Can you work these out from the model? Positions are in its coordinate system, mm. A direction names the side the tool comes from. Give positions to 0.01 mm unless a question says otherwise; leave off trailing zeros. Loops run counter-clockwise (first coordinate to the right, second up) from the corner with the lowest first, then second, coordinate; pieces in that order, holes last.
from build123d import *

# Parameters (mm, degrees)
CYLINDER870_R               = 1.5
CYLINDER870_DEPTH           = 20
CYLINDER865_R               = 1.5
CYLINDER865_DEPTH           = 20
CYLINDER862_R               = 1.5
CYLINDER862_DEPTH           = 20
CYLINDER868_R               = 1.5
CYLINDER868_DEPTH           = 20
BOX131_W                    = 6
BOX131_H                    = 2
BOX131_DEPTH                = 6
BOX130_W                    = 6
BOX130_H                    = 2
BOX130_DEPTH                = 6
BOX133_W                    = 6
BOX133_H                    = 2
BOX133_DEPTH                = 6
BOX132_W                    = 6
BOX132_H                    = 2
BOX132_DEPTH                = 6
CYLINDER872_R               = 4
CYLINDER872_DEPTH           = 20
CYLINDER872_PLACEMENT_ANGLE = 45
CYLINDER871_R               = 4
CYLINDER871_DEPTH           = 20
CYLINDER871_PLACEMENT_ANGLE = 45
CYLINDER863_R               = 10
CYLINDER863_DEPTH           = 40
CYLINDER908_R               = 10
CYLINDER908_DEPTH           = 40
CYLINDER864_R               = 52
CYLINDER864_DEPTH           = 10
BOX129_W                    = 108
BOX129_H                    = 36
BOX129_DEPTH                = 10
FILLET013_R                 = 12


with BuildPart() as obj1:
    # Cylinder870 → Cylinder870 (new body)
    with BuildSketch(Plane(origin=(20, -40, -5), x_dir=(1, 0, 0), z_dir=(0, -1, 0))):
        Circle(CYLINDER870_R)
    extrude(amount=CYLINDER870_DEPTH)


with BuildPart() as obj2:
    # Cylinder865 → Cylinder865 (new body)
    with BuildSketch(Plane(origin=(51, -40, 7), x_dir=(1, 0, 0), z_dir=(0, -1, 0))):
        Circle(CYLINDER865_R)
    extrude(amount=CYLINDER865_DEPTH)


with BuildPart() as obj3:
    # Cylinder862 → Cylinder862 (new body)
    with BuildSketch(Plane(origin=(-51, -40, 7), x_dir=(1, 0, 0), z_dir=(0, -1, 0))):
        Circle(CYLINDER862_R)
    extrude(amount=CYLINDER862_DEPTH)


with BuildPart() as compound261:
    # Cylinder868 → Cylinder868 (new body)
    with BuildSketch(Plane(origin=(-20, -40, -5), x_dir=(1, 0, 0), z_dir=(0, -1, 0))):
        Circle(CYLINDER868_R)
    extrude(amount=CYLINDER868_DEPTH)

    # Compound261: union obj1, obj2, obj3
    add(obj1.part)
    add(obj2.part)
    add(obj3.part)


with BuildPart() as krychle131:
    # Box131 → Box131 (new body)
    with BuildSketch(Plane(origin=(17, -47, -8), x_dir=(1, 0, 0), z_dir=(0, 0, 1))):
        with Locations((3, 1)):
            Rectangle(BOX131_W, BOX131_H)
    extrude(amount=BOX131_DEPTH)


with BuildPart() as krychle130:
    # Box130 → Box130 (new body)
    with BuildSketch(Plane(origin=(48, -45, 4), x_dir=(1, 0, 0), z_dir=(0, 0, 1))):
        with Locations((3, 1)):
            Rectangle(BOX130_W, BOX130_H)
    extrude(amount=BOX130_DEPTH)


with BuildPart() as krychle133:
    # Box133 → Box133 (new body)
    with BuildSketch(Plane(origin=(-54, -45, 4), x_dir=(1, 0, 0), z_dir=(0, 0, 1))):
        with Locations((3, 1)):
            Rectangle(BOX133_W, BOX133_H)
    extrude(amount=BOX133_DEPTH)


with BuildPart() as compound258:
    # Box132 → Box132 (new body)
    with BuildSketch(Plane(origin=(-23, -47, -8), x_dir=(1, 0, 0), z_dir=(0, 0, 1))):
        with Locations((3, 1)):
            Rectangle(BOX132_W, BOX132_H)
    extrude(amount=BOX132_DEPTH)

    # Compound258: union Krychle131, Krychle130, Krychle133
    add(krychle131.part)
    add(krychle130.part)
    add(krychle133.part)


with BuildPart() as obj4:
    # Cylinder872 → Cylinder872 (new body)
    with BuildSketch(Plane.XY):
        Circle(CYLINDER872_R)
    extrude(amount=CYLINDER872_DEPTH)


with BuildPart() as obj4_1:
    # Cylinder872 placement: moved
    add(obj4.part.moved(Location((39.6, -39.6, -10))).rotate(Axis((39.6, -39.6, -10), (0, 0, 1)), CYLINDER872_PLACEMENT_ANGLE))


with BuildPart() as compound259:
    # Cylinder871 → Cylinder871 (new body)
    with BuildSketch(Plane.XY):
        Circle(CYLINDER871_R)
    extrude(amount=CYLINDER871_DEPTH)


with BuildPart() as compound259_1:
    # Cylinder871 placement: moved
    add(compound259.part.moved(Location((-39.6, -39.6, -10))).rotate(Axis((-39.6, -39.6, -10), (0, 0, -1)), CYLINDER871_PLACEMENT_ANGLE))

    # Compound259: union obj4
    add(obj4_1.part)


with BuildPart() as obj5:
    # Cylinder863 → Cylinder863 (new body)
    with BuildSketch(Plane(origin=(-59, -17, 0), x_dir=(1, 0, 0), z_dir=(0, 0, 1))):
        Circle(CYLINDER863_R)
    extrude(amount=CYLINDER863_DEPTH)


with BuildPart() as compound260:
    # Cylinder908 → Cylinder908 (new body)
    with BuildSketch(Plane(origin=(59, -17, 0), x_dir=(1, 0, 0), z_dir=(0, 0, 1))):
        Circle(CYLINDER908_R)
    extrude(amount=CYLINDER908_DEPTH)

    # Compound260: union obj5
    add(obj5.part)


with BuildPart() as obj6:
    # Cylinder864 → Cylinder864 (new body)
    with BuildSketch(Plane.XY.offset(20)):
        Circle(CYLINDER864_R)
    extrude(amount=CYLINDER864_DEPTH)


with BuildPart() as fillet013:
    # Box129 → Box129 (new body)
    with BuildSketch(Plane(origin=(-54, -53, 20), x_dir=(1, 0, 0), z_dir=(0, 0, 1))):
        with Locations((54, 18)):
            Rectangle(BOX129_W, BOX129_H)
    extrude(amount=BOX129_DEPTH)

    # Cut147: cut obj6
    add(obj6.part, mode=Mode.SUBTRACT)


with BuildPart() as fillet013_1:
    # Cut147 placement: moved
    add(fillet013.part.moved(Location((0, 0, -20))))

    # Cut146: cut Compound260
    add(compound260.part, mode=Mode.SUBTRACT)

    # Cut149: cut Compound259
    add(compound259_1.part, mode=Mode.SUBTRACT)

    # Cut148: cut Compound258
    add(compound258.part, mode=Mode.SUBTRACT)

    # Cut150: cut Compound261
    add(compound261.part, mode=Mode.SUBTRACT)

    # Fillet013
    fillet013_edges = [fillet013_1.edges().sort_by_distance(p)[0] for p in [
        (-54, -25.660254, 5),
        (54, -25.660254, 5),
    ]]
    fillet(fillet013_edges, radius=FILLET013_R)


solid = fillet013_1.part
(1) Will these pins go through, and if not, where does the flat tip stop? P1, Ø10.5, axis at x = 39.6, y = -39.6, coming from the -Z side; P2, Ø2.5, axis at x = -51, z = 7, coming from the +Y side; P3, Ø1.5, axis at x = -38.5, z = 1.5, coming from the +Y side; P4, Ø1, axis at y = -44, z = 8, coming from the +X side.
Returned:
P1: stops at z = 0
P2: stops at y = -20.8
P3: stops at y = -34.11
P4: stops at x = 48
(2) Suppose I cut it at A-A on y = -48.5. List the corners of the cut face in (x, z) for me (3 decimals).
Returned:
outline: (-54, 0) - (-18.755, 0) - (-18.755, 10) - (-54, 10) - close; (18.755, 0) - (54, 0) - (54, 10) - (18.755, 10) - close; hole circle Ø3 at (-51, 7); hole circle Ø3 at (51, 7)
(3) Please list where these lines run through material, in increasing order: probe 1 along X at (y, z) = (-39.6, 2.75); probe 2 along X at (y, z) = (-47.5, 7); probe 3 along X at (y, z) = (-21.5, 8.5).
Returned:
probe 1: x = -54 to -43.6, -35.6 to -33.7, 33.7 to 35.6, 43.6 to 54
probe 2: x = -54 to -52.5, -49.5 to -21.16, 21.16 to 49.5, 52.5 to 54
probe 3: x = -50.07 to -47.35, 47.35 to 50.07
(4) Suppose I cut it at B-B on z = 7. Give the number of separate pieces and of enclosed holes in the cut face, plus the area to 3 significant figures.
Returned:
separate pieces: 3
enclosed holes: 2
area: 1,120 mm2
(5) Suppose I cut it at C-C on x = 38. List the corners of the cut face in (y, z) for me.
Returned:
outline: (-53, 0) - (-43.27, 0) - (-43.27, 10) - (-53, 10) - close; (-35.93, 0) - (-35.5, 0) - (-35.5, 10) - (-35.93, 10) - close
(6) Which directions (+Z, -Z, +X, -X, +Y, -Y) give clear straight access to the entire face, cutting with the end or side of a thin tool? Please do faces 1 (the flat face through (-52.4, -45, 5.6)), 2 (the cylindrical face through (49.8, -48.9, 6.1)), 3 (the flat face through (54, -42, 5)), 4 (the cylindrical face through (-0.895, -51.992, 4.93)), 5 (the flat face through (48, -44, 7)).
Returned:
face 1: +Z, -X
face 2: -Y
face 3: +Z, -Z, +X, +Y, -Y
face 4: +Z, -Z, +Y
face 5: +Z, +X
(7) Thinking about a two-plate mould opening in Z: for faces 6 (the flat face through (-51, -44, 4)), 7 (the flat face through (-13, -51, 0)), 8 (the cylindrical face through (-52.2, -41.5, 6.1)), 9 (the cylindrical face through (49.636, -20.51, 4.93)), which applies, pulls with the +Z half, pulls with the -Z half, needs draft (parallel to the pull), parting line crosses it, or undercut?
Returned:
face 6: pulls with the +Z half
face 7: pulls with the -Z half
face 8: undercut
face 9: needs draft
(8) Suppose I cut it at D-D on y = -30. List the corners of the cut face in (x, z) for me.
Returned:
outline: (-53.96, 0) - (-42.47, 0) - (-42.47, 10) - (-53.96, 10) - close; (42.47, 0) - (53.96, 0) - (53.96, 10) - (42.47, 10) - close
